Autodesk Inventor part; units mm, degrees
ref_plane "YZ Plane" through (0, 0, 0) normal (1, 0, 0) x (0, 1, 0)
ref_plane "XZ Plane" through (0, 0, 0) normal (0, 1, 0) x (-1, 0, 0)
ref_plane "XY Plane" through (0, 0, 0) normal (0, 0, 1) x (1, 0, 0)
sketch "Esquisse2" plane through (0, 0, 0) normal (1, 0, 0) x (0, 1, 0)
  line L0 (6.25, -10) -> (6.25, -11)
  line L1 (6.25, -11) -> (9.5, -21)
  line L2 (9.5, -21) -> (9.5, -31)
  line L3 (0, -252.0623) -> (0, 0)
  line L4 (9.5, -31) -> (12.5, -31)
  line L5 (12.5, -31) -> (12.5, 0)
  line L6 (6.25, -10) -> (7.75, -10)
  line L7 (12.5, 0) -> (7.75, 0)
  line L8 (7.75, 0) -> (7.75, -10)
  dimension "d1" = 10
  dimension "d4" = 12.5
  dimension "d6" = 3
  dimension "d8" = 1.5
  dimension "d11" = 19
  dimension "d12" = 20
  dimension "d15" = 25
  dimension "d16" = 1
  dimension "d17" = 10
  dimension "d22" = 15.5
revolve "Révolution1" add sketch "Esquisse2" angle 360 about axis through (0, 0, -252.0623) along (0, 0, 1)
thread "Filetage3"
chamfer "Chanfrein1" distance 0.5 angle 45 1 edges at (0, -7.75, 0)
sketch "Esquisse7" plane through (0, 0, -31) normal (0, 0, -1) x (-1, 0, 0)
  line L0 (-11.6247, -16) -> (-18.8091, 6.1115)
  line L1 (-18.8091, 6.1115) -> (0, 19.7771)
  line L2 (0, 19.7771) -> (18.8091, 6.1115)
  line L3 (18.8091, 6.1115) -> (11.6247, -16)
  line L4 (11.6247, -16) -> (-11.6247, -16)
  circle A0 centre (0, 0) radius 12.5
  circle A1 centre (0, 0) radius 9.5
  dimension "d44" = 16
extrude "Extrusion5" add sketch "Esquisse7" against normal up to surface (31 mm away) contours L0 L1 L2 L3 L4
sketch "Esquisse8" plane through (11.6247, -16, 0) normal (0.9511, -0.309, 0) x (0, 0, -1)
  line L0 (21, 2.1247) -> (21, 21.1247)
  line L1 (11, 5.3747) -> (11, 17.8747)
  line L2 (10, 5.3747) -> (10, 17.8747)
  point P0 (0, 11.6247)
  point P1 (11, 11.6247)
  point P2 (11, 11.6247)
hole "Perçage2" at (15.2169, -4.9443, -11) direction (-0.9511, 0.309, 0) diameter 4.134 depth 7 tip angle 118
mirror "Symétrie1" about plane through (0, 0, 0) normal (1, 0, 0) of "Perçage2"
chamfer "Chanfrein2" distance 4 angle 45 1 edges at (0, -9.5, -31)
properties part number "ammo_blocker"
Input: part model. Units: mm. Frame: model coordinates. A direction names the side the tool comes from. Coordinates: 2 decimals unless noted, no trailing zeros. Write each loop counter-clockwise with the first axis right and the second up, starting at its lowest first coordinate (ties: lowest second). Pieces come first, ordered by that corner, then holes.
1) Section A-A on z = -28. Output: boundary loops of the cut face in (x, y).
2) Set-up query: faces 4 (the flat face through (9, -2, 0)), 5 (the cylindrical face through (7.684, -1.009, -5.316)), 6 (the cylindrical face through (-8.43, 4.38, -24.04)), 7 (the conical face through (-7.55, -2.57, -11.34)). Return all of +Z, -Z, +X, -X, +Y, -Y with unobstructed straight access to the full face (end or side cutting, diameter ignored); none if empty.
3) Section B-B on y = 0. Output: boundary loops of the cut face in (x, z), and give its area (3 significant figures).
4) Pin query (flat end, axial travel): pin 1 Ø1 at (y, z) = (9.5, -15.5) entering from +X; pin 2 Ø1.5 at (x, y) = (-4, -4.5) entering from +Z; pin 3 Ø4 at (y, z) = (-12, -8.5) entering from -X. Return the tip coordinate at first contact, or that it passes through.
5) Material intervals for line 1 along Y through (x, z) = (0, -4.75); line 2 along Y through (x, z) = (0, -25); line 3 along X through (y, z) = (-1.5, -28), sorted ascending.
6) Mould query, pull axis Z, two halves, no side actions, for faces 1 (the cylindrical face through (12.086, -3.095, -12.909)), 2 (the flat face through (-9.27, 13.04, -15.72)), 3 (the flat face through (-6.4, 0.5, -10)). Classes: pulls with the +Z half, pulls with the -Z half, needs draft (parallel to the pull), parting line crosses it, or undercut.
7) Section C-C on z = -17. Output: boundary loops of the cut face in (x, y), and give its area (3 significant figures).
Check result:
1. outline: (-18.81, 6.11) - (-11.62, -16) - (11.62, -16) - (18.81, 6.11) - (0, 19.78) - close; hole circle Ø21 at (0, 0)
2. face 4: +Z, +X, -X, +Y, -Y
2. face 5: +Z
2. face 6: -Z
2. face 7: none
3. outline: (-16.82, -31) - (-13.5, -31) - (-9.5, -27) - (-9.5, -21) - (-6.25, -11) - (-6.25, -10) - (-7.75, -10) - (-7.75, -0.5) - (-8.25, 0) - (-16.82, 0) - close; (6.25, -11) - (9.5, -21) - (9.5, -27) - (13.5, -31) - (16.82, -31) - (16.82, 0) - (8.25, 0) - (7.75, -0.5) - (7.75, -10) - (6.25, -10) - close
3. area: 512 mm2
4. pin 1: stops at x = 14.83
4. pin 2: stops at z = -10
4. pin 3: stops at x = -13.57
5. line 1: y = -16 to -7.75, 7.75 to 19.78
5. line 2: y = -16 to -9.5, 9.5 to 19.78
5. line 3: x = -16.34 to -10.39, 10.39 to 16.34
6. face 1: undercut
6. face 2: needs draft
6. face 3: pulls with the +Z half
7. outline: (-18.81, 6.11) - (-11.62, -16) - (11.62, -16) - (18.81, 6.11) - (0, 19.78) - close; hole circle Ø16.4 at (0, 0)
7. area: 719 mm2
